Work out the finished part from the listing and answer in its coordinate system (mm). A direction names the side the tool comes from. Round coordinates to 2 decimals unless told otherwise and drop trailing zeros. Loops run counter-clockwise (first coordinate to the right, second up) from the corner with the lowest first, then second, coordinate; pieces in that order, holes last.
from build123d import *

# Parameters (mm, degrees)
F0_R     = 11
F1_DEPTH = 10
F2_COUNT = 3
F4_R     = 10.5
F5_DEPTH = 25
F6_R     = 50
F7_T     = -2


with BuildPart() as f1:
    # F0 (on Top) → F1 (new body)
    with BuildSketch(Plane.XY):
        with BuildLine():
            Line((-12.5, 27.2717802866), (-37.2916666667, 15.9085385005))
            ThreePointArc((-37.2916666667, 15.9085385005), (-47.5, 0), (-37.2916666667, -15.9085385005))
            Line((-37.2916666667, -15.9085385005), (-12.5, -27.2717802866))
            ThreePointArc((-12.5, -27.2717802866), (30, 0), (-12.5, 27.2717802866))
        make_face()
        Circle(F0_R, mode=Mode.SUBTRACT)
    extrude(amount=F1_DEPTH)


with BuildPart() as f2_1:
    # F2: instance of F1
    add(f1.part.rotate(Axis((0, 0, 0), (0, 0, -1)), 1 * 360 / F2_COUNT))


with BuildPart() as f2_2:
    # F2: instance of F1
    add(f1.part.rotate(Axis((0, 0, 0), (0, 0, -1)), 2 * 360 / F2_COUNT))


with BuildPart() as f1_1:
    add(f1.part)

    # F3: union F2_1, F2_2
    add(f2_1.part)
    add(f2_2.part)

    # F4 (on face) → F5 (cut)
    with BuildSketch(Plane.XY.offset(10)):
        with Locations((15, 25.9807621135)):
            Circle(F4_R)
        with Locations((15, -25.9807621135)):
            Circle(F4_R)
        with Locations((-30, 0)):
            Circle(F4_R)
    extrude(amount=-F5_DEPTH, mode=Mode.SUBTRACT)

    # F6
    f6_edges = [f1_1.edges().sort_by_distance(p)[0] for p in [
        (-15.066264, -26.095535, 5),
        (-15.066264, 26.095535, 5),
        (30.132528, 0, 5),
    ]]
    fillet(f6_edges, radius=F6_R)

    # F7
    f7_openings = [f1_1.faces().sort_by_distance(p)[0] for p in [
        (-27.825176, 18.947668, 0),
    ]]
    offset(amount=F7_T, openings=f7_openings)


solid = f1_1.part
Item 1: Straight lines are drawn through the part: line 1 (Y direction, x = 15, z = 3.5); line 2 (Y direction, x = 18, z = 6); line 3 (Y direction, x = 0, z = 3.25). For each, find the intervals that lie inside material, in ascending order.
Item 2: Each of these flat-tipped pins is pushed along its axis until it touches: P1, Ø5, axis at y = -11, z = 2.5, coming from the +X side; P2, Ø19, axis at x = 15, y = -25.98, coming from the +Z side; P3, Ø6, axis at y = -9.5, z = 8, coming from the +X side; P4, Ø5, axis at x = -1.5, z = 6.5, coming from the -Y side. Where does it stop, or does it pass through?
Item 3: Section A-A, the plane y = 0 is taken. Give the vertices of the cut face in (x, z), plus the area to 3 significant figures.
Item 4: Section B-B, the plane x = 15 is taken. Give the vertices of the cut face in (y, z), plus the area to 3 significant figures.
Item 5: Determine the mould class of faces 1 (the face through (-1.91, 32.984, 3.944)), 2 (the face through (-15.12, -26.32, 4.93)), 3 (the face through (26, -25, 0)), 4 (the face through (31.51, -14.65, 4.93)) for opening direction X: pulls with the +X half, pulls with the -X half, needs draft (parallel to the pull), parting line crosses it, or undercut.
Item 6: Section C-C, the plane z = 3.75 is taken. State how many separate pieces and enclosed holes the cut face has, plus the area to 3 significant figures.
Item 7: For faces 5 (the face through (-27.61, -18.146, 3.944)), 6 (the face through (-28.19, 20.08, 4.93)), determine the directions among +Z, -Z, +X, -X, +Y, -Y from which every point of the face is accessible in a straight line to the end or side of a thin tool.
Item 8: Section D-D, the plane x = 0 is taken. Give the vertices of the cut face in (y, z), plus the area to 3 significant figures.
Answer below:
1. line 1: y = -43.48 to -41.48, -38.48 to -36.48, -15.48 to -13.48, 13.48 to 15.48, 36.48 to 38.48, 41.48 to 43.48
1. line 2: y = -43.22 to -41.19, -38.12 to -36.04, -15.92 to -13.85, 13.85 to 15.92, 36.04 to 38.12, 41.19 to 43.22
1. line 3: y = -36.79 to -34.34, -13 to -11, 11 to 13, 34.34 to 36.79
2. P1: stops at x = 31.4
2. P2: passes through
2. P3: stops at x = 31.31
2. P4: stops at y = -37.5
3. outline: (-47.5, 0) - (-45.5, 0) - (-45.5, 8) - (-42.5, 8) - (-42.5, 0) - (-40.5, 0) - (-40.5, 10) - (-47.5, 10) - close; (-19.5, 0) - (-17.5, 0) - (-17.5, 8) - (-13, 8) - (-13, 0) - (-11, 0) - (-11, 10) - (-19.5, 10) - close; (11, 0) - (13, 0) - (13, 8) - (28.35, 8) - (28.35, 0) - (30.35, 0) - (30.35, 10) - (11, 10) - close
3. area: 166 mm2
4. outline: (-43.48, 0) - (-41.48, 0) - (-41.48, 8) - (-38.48, 8) - (-38.48, 0) - (-36.48, 0) - (-36.48, 10) - (-43.48, 10) - close; (-15.48, 0) - (-13.48, 0) - (-13.48, 8) - (13.48, 8) - (13.48, 0) - (15.48, 0) - (15.48, 10) - (-15.48, 10) - close; (36.48, 0) - (38.48, 0) - (38.48, 8) - (41.48, 8) - (41.48, 0) - (43.48, 0) - (43.48, 10) - (36.48, 10) - close
4. area: 186 mm2
5. face 1: undercut
5. face 2: pulls with the -X half
5. face 3: needs draft
5. face 4: pulls with the +X half
6. separate pieces: 5
6. enclosed holes: 5
6. area: 1,100 mm2
7. face 5: -Z
7. face 6: +Z, -Z, -X, +Y
8. outline: (-36.79, 0) - (-34.34, 0) - (-34.34, 8) - (-13, 8) - (-13, 0) - (-11, 0) - (-11, 10) - (-36.79, 10) - close; (11, 0) - (13, 0) - (13, 8) - (34.34, 8) - (34.34, 0) - (36.79, 0) - (36.79, 10) - (11, 10) - close
8. area: 174 mm2
